Input: part model. Units: mm. Frame: model coordinates. A direction names the side the tool comes from. Coordinates: 2 decimals unless noted, no trailing zeros. Order: outer loops, then holes, each group sorted by start corner. A loop starts at its lowest first (then second) coordinate and runs counter-clockwise, first axis right, second up.
from build123d import *

# Parameters (mm, degrees)
F0_R     = 1.5875
F1_DEPTH = 25.4


with BuildPart() as f1:
    # F0 (on Front) → F1 (new body)
    with BuildSketch(Plane.XZ):
        Polygon((0, 25.4), (0, 0), (25.4, 0), (25.4, 5.125011), (22.046786, 5.125011), (5.55021, 5.125011), (5.55021, 21.746561), (17.73518, 21.746561), (17.73518, 18.43475), (25.4, 18.43475), (25.4, 25.4), align=None)
        with Locations((22.151161, 22.445666)):
            Circle(F0_R, mode=Mode.SUBTRACT)
        Polygon((22.046786, 5.125011), (25.4, 5.125011), (25.4, 9.061695), (25.4, 10.373922), (22.046786, 10.373922), align=None)
        Polygon((25.4, 10.373922), (25.4, 13.935683), (11.111556, 13.935683), (11.111556, 10.373922), (22.046786, 10.373922), align=None)
    extrude(amount=F1_DEPTH)


solid = f1.part
Item 1: Draft query along X for faces 4 (the face through (25.4, -13, 7)), 5 (the face through (17, -13, 10.374)), 6 (the face through (13, 0, 13)). Return one class per face: pulls with the +X half, pulls with the -X half, needs draft (parallel to the pull), parting line crosses it, or undercut.
Response values:
face 4: pulls with the +X half
face 5: undercut
face 6: needs draft
Item 2: Cut plane B-B on z = 6.5. Return loops of the section in (x, y), then the cut area to 3 significant figures.
Response values:
outline: (0, -25.4) - (5.55, -25.4) - (5.55, 0) - (0, 0) - close; (22.05, -25.4) - (25.4, -25.4) - (25.4, 0) - (22.05, 0) - close
area: 226 mm2
Item 3: Ray query, probe 1 along Z at (x, y) = (11.25, -17); probe 2 along X at (y, z) = (-8, 6.75); probe 3 along Z at (x, y) = (6.75, -9.25). Return the intervals inside material, ascending.
Response values:
probe 1: z = 0 to 5.13, 10.37 to 13.94, 21.75 to 25.4
probe 2: x = 0 to 5.55, 22.05 to 25.4
probe 3: z = 0 to 5.13, 21.75 to 25.4
Item 4: Cut plane D-D on y = -3.25. Return loops of the section in (x, z) (1 decimal).
Response values:
outline: (0, 0) - (25.4, 0) - (25.4, 13.9) - (11.1, 13.9) - (11.1, 10.4) - (22, 10.4) - (22, 5.1) - (5.6, 5.1) - (5.6, 21.7) - (17.7, 21.7) - (17.7, 18.4) - (25.4, 18.4) - (25.4, 25.4) - (0, 25.4) - close; hole circle Ø3.2 at (22.2, 22.4)
Item 5: Cut plane C-C on x = 7.75. Return loops of the section in (y, z).
Response values:
outline: (-25.4, 0) - (0, 0) - (0, 5.13) - (-25.4, 5.13) - close; (-25.4, 21.75) - (0, 21.75) - (0, 25.4) - (-25.4, 25.4) - close
Item 6: Access query for faces 1 (the face through (18, -13, 13.936)), 2 (the face through (11.112, -13, 12)), 3 (the face through (13, -25.4, 13)). Directions: +Z, -Z, +X, -X, +Y, -Y. A direction counts if a zero-diameter tool reaches every point of the face in a straight line with its end or side. Return the directions, or none.
Response values:
face 1: +X, +Y, -Y
face 2: +Y, -Y
face 3: +Z, -Z, +X, -X, -Y
Item 7: Cut plane A-A on x = 19.5. Return loops of the section in (y, z), then the cut area to 3 significant figures.
Response values:
outline: (-25.4, 0) - (0, 0) - (0, 5.13) - (-25.4, 5.13) - close; (-25.4, 10.37) - (0, 10.37) - (0, 13.94) - (-25.4, 13.94) - close; (-25.4, 18.43) - (0, 18.43) - (0, 25.4) - (-25.4, 25.4) - close
area: 398 mm2
